Design review of the part built by this model. Coordinates are the model's own, in mm. Coordinates: 2 decimals unless noted, no trailing zeros. Write each loop counter-clockwise with the first axis right and the second up, starting at its lowest first coordinate (ties: lowest second). Pieces come first, ordered by that corner, then holes. Notation, with made-up numbers: (-20, -34.75) -> (-2, -34.75) arc R37 cw to (-2, 1.25) -> close; hole circle Ø11 at (50.5, -17.75). An arc over 180 degrees is marked (long way). Answer in a Markdown table with one row per item. Add a question column.
Item 1: Take a section at A-A, the plane x = 5.5. Write out the cut boundary in (y, z) (3 decimals).
Item 2: To check wall thickness, follow line 1 (X direction, y = 1.5, z = 361.5) (3 decimals); line 2 (X direction, y = -20, z = 117.5). State the ranges of each line that lie inside material, in increasing order.
Item 3: Take a section at C-C, the plane y = 10.5. Write out the cut boundary in (x, z) (3 decimals), and give its area (3 significant figures).
Item 4: Take a section at B-B, the plane z = 455. Write out the cut boundary in (x, y) (3 decimals).
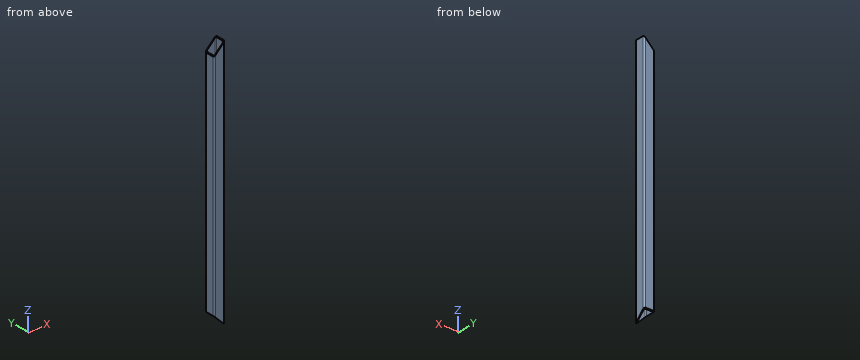
Autodesk Inventor part; units mm, degrees
ref_plane "Plano inicial" through (0, 0, 1.8599) normal (0, 0, 1) x (1, 0, 0)
ref_plane "Plano final" through (0, 0, 1175.4) normal (0, 0, 1) x (1, 0, 0)
ref_plane "Plano de trabajo4" through (25.4, 0, 1175.4) normal (-0.7071, 0, 0.7071) x (0.7071, 0, 0.7071)
ref_plane "Plano inicial" through (0, 0, 1.8599) normal (0, 0, 1) x (1, 0, 0)
ref_plane "Plano final" through (0, 0, 1175.4) normal (0, 0, 1) x (1, 0, 0)
sketch "Boceto" plane through (0, 0, 0) normal (0, 0, 1) x (1, 0, 0)
  line L0 (-25.4, -19.05) -> (-25.4, 19.05)
  line L1 (-19.05, 25.4) -> (19.05, 25.4)
  line L2 (25.4, 19.05) -> (25.4, -19.05)
  line L3 (19.05, -25.4) -> (-19.05, -25.4)
  arc A0 (-25.4, -19.05) -> (-19.05, -25.4) centre (-19.05, -19.05) ccw
  arc A1 (-19.05, 25.4) -> (-25.4, 19.05) centre (-19.05, 19.05) ccw
  arc A2 (25.4, 19.05) -> (19.05, 25.4) centre (19.05, 19.05) ccw
  arc A3 (19.05, -25.4) -> (25.4, -19.05) centre (19.05, -19.05) ccw
  arc A4 (-19.05, 22.225) -> (-22.225, 19.05) centre (-19.05, 19.05) ccw
  line L4 (-19.05, 22.225) -> (19.05, 22.225)
  arc A5 (22.225, 19.05) -> (19.05, 22.225) centre (19.05, 19.05) ccw
  line L5 (22.225, 19.05) -> (22.225, -19.05)
  arc A6 (19.05, -22.225) -> (22.225, -19.05) centre (19.05, -19.05) ccw
  line L6 (19.05, -22.225) -> (-19.05, -22.225)
  arc A7 (-22.225, -19.05) -> (-19.05, -22.225) centre (-19.05, -19.05) ccw
  line L7 (-22.225, -19.05) -> (-22.225, 19.05)
  line L8 (0, 37.4012) -> (0, -37.4012) construction
  line L9 (-37.4012, 0) -> (37.4012, 0) construction
  dimension "d10" = 50.8
  dimension "d11" = 50.8
  dimension "d12" = 3.175
  dimension "d15" = 25.4
  dimension "d16" = 25.4
  dimension "d17" = 6.35
extrude "Cuerpo" add sketch "Boceto" along normal up to surface (1173.5401 mm away) from surface at 1.8599
sketch "Sketch3" plane through (0, 0, 0) normal (0, 0, 1) x (1, 0, 0)
  line L0 (0, 0) -> (10, 0)
ref_plane "Work Plane3" through (0, 0, 0) normal (0, -1, 0) x (1, 0, 0)
ref_plane "Plano de trabajo4" through (25.4, 0, 1175.4) normal (-0.7071, 0, 0.7071) x (0.7071, 0, 0.7071)
split "Dividir1" plane through (25.4, 0, 1175.4) removes the side toward (-0.7071, 0, 0.7071)
ref_plane "Plano de trabajo5" through (0, -25.4, 0) normal (0, 0.7071, -0.7071) x (1, 0, 0)
split "Dividir2" plane through (0, -25.4, 0) removes the side toward (0, 0.7071, -0.7071)
ref_plane "Plano de trabajo6" through (25.4, 0, 0) normal (-0.7071, 0, -0.7071) x (-0.7071, 0, 0.7071)
split "Dividir3" plane through (25.4, 0, 0) removes the side toward (-0.7071, 0, -0.7071)
sketch "Sketch4" plane through (0, 0, 0) normal (0, -1, 0) x (1, 0, 0)
  line L0 (-2, 1.8599) -> (12, 1.8599)
  line L1 (-2, 1175.4) -> (12, 1175.4)
  dimension "d19" = 1173.5401
equation "\"d10\" = G_H"
equation "\"d11\" = G_W"
equation "\"d12\" = G_T"
equation "\"d15\" = 0.5 * d10"
equation "\"d16\" = 0.5 * d11"
equation "\"d17\" = G_IR"
equation "\"d3\" = G_L"
equation "\"G_W\" = 50.8"
equation "\"G_H\" = 50.8"
equation "\"G_T\" = 3.175"
equation "\"G_IR\" = 6.35"
equation "\"G_L\" = d19"
equation "\"G_OFFSET_START\" = -1.85987"
equation "\"G_OFFSET_END\" = 25.4"
equation "\"d13\" = -G_OFFSET_START"
equation "\"d14\" = G_OFFSET_END + B_L"
equation "\"B_L\" = 1150"
properties part number "AISC - 2 x 2 x 1/8 - 46,202" material "Acero, suave"
Answers:
| question | item | result |
|---|---|---|
| 1 | outline | (-25.4, 19.9) -> (-22.225, 19.9) -> (-22.225, 1155.5) -> (-25.4, 1155.5) -> close; (22.225, 47.625) -> (25.4, 50.8) -> (25.4, 1155.5) -> (22.225, 1155.5) -> close |
| 2 | line 1 | x = -25.4 to -22.225, 22.225 to 25.4 |
| 2 | line 2 | x = -25.33 to -22.08, 22.08 to 25.33 |
| 3 | outline | (-25.4, 50.8) -> (-22.225, 47.625) -> (-22.225, 1127.775) -> (-25.4, 1124.6) -> close; (22.225, 35.9) -> (25.4, 35.9) -> (25.4, 1175.4) -> (22.225, 1172.225) -> close |
| 3 | area | 7,030 mm^2 |
| 4 | outline | (-25.4, -19.05) arc R6.35 ccw to (-19.05, -25.4) -> (19.05, -25.4) arc R6.35 ccw to (25.4, -19.05) -> (25.4, 19.05) arc R6.35 ccw to (19.05, 25.4) -> (-19.05, 25.4) arc R6.35 ccw to (-25.4, 19.05) -> close; hole (-22.225, -19.05) arc R3.175 ccw to (-19.05, -22.225) -> (19.05, -22.225) arc R3.175 ccw to (22.225, -19.05) -> (22.225, 19.05) arc R3.175 ccw to (19.05, 22.225) -> (-19.05, 22.225) arc R3.175 ccw to (-22.225, 19.05) -> close |
